Verification items for this drawing (mm, ordinates from the low corner). A direction names the side the tool comes from. Round coordinates to 2 decimals unless told otherwise and drop trailing zeros. Loops run counter-clockwise (first coordinate to the right, second up) from the corner with the lowest first, then second, coordinate; pieces in that order, holes last. Notation, with made-up numbers: (-5, 15.25) - (5, 15.25) arc R25 ccw to (5, 37.25) - close; hole circle Ø11 at (66.25, -6). An arc over 180 degrees is marked (long way). Answer in a Markdown table with one row per item. Add a question column.
(1) Gauge pin test, flat ends, axial feed: pin 1 (0.9 mm diameter, centred on y = 3.5, z = 3, fed in from +X); pin 2 (1.6 mm diameter, centred on x = 0.5, y = 2.5, fed in from +Z); pin 3 (1.8 mm diameter, centred on x = 3, y = 3, fed in from -Z); pin 4 (1 mm diameter, centred on x = 7.5, z = 2.5, fed in from -Y). Record the tip position at first contact, or that the pin passes through.
(2) Cross-section at D-D on x = 4. Enter the section's corners in (y, z), then the cut area to 3 significant figures.
(3) Cross-section at A-A on z = 2.75. Enter the section's corners in (x, y) (3 decimals).
(4) Access from +Z, -Z, +X, -X, +Y, -Y to the whole of each face (thin tool, end or side, straight path). Record for the marked faces 1, 2, 3, 4 and 5.
(5) Thickness scan on line 1 along X through (y, z) = (1.5, 3.25) (3 decimals); line 2 along X through (y, z) = (4.2, 3.5); line 3 along Z through (x, y) = (0.75, 4.35). Record the ranges inside material, lowest first.
(6) Cross-section at C-C on x = 5. Enter the section's corners in (y, z).
(7) Cross-section at B-B on x = 1.1. Enter the section's corners in (y, z) (3 decimals).
(8) Mould release check, pull along X, two halves, no side actions. Record for the marked faces 6, 7, 8 and 9: +X half, -X half, draft (parallel to the pull), parting line (faces both ways), or undercut.
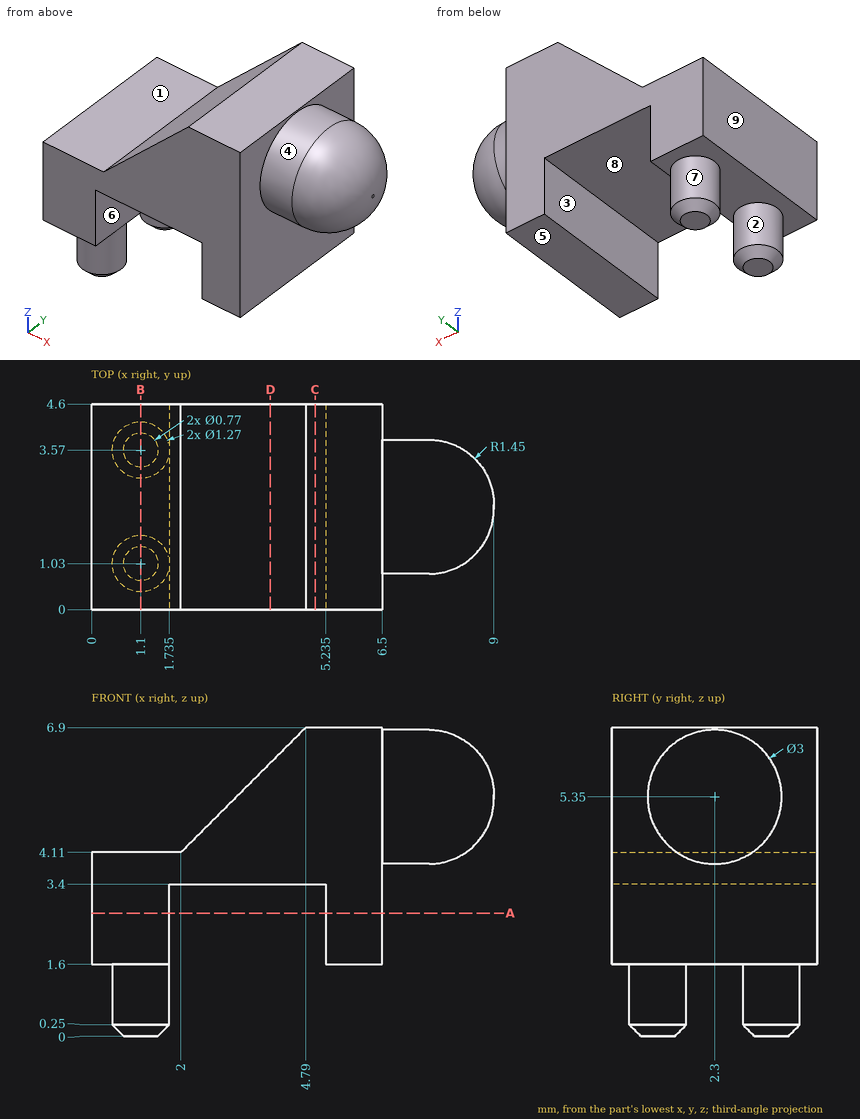
Answers:
| question | item | result |
|---|---|---|
| 1 | pin 1 | stops at x = 6.5 |
| 1 | pin 2 | stops at z = 4.11 |
| 1 | pin 3 | stops at z = 3.4 |
| 1 | pin 4 | passes through |
| 2 | outline | (0, 3.4) - (4.6, 3.4) - (4.6, 6.11) - (0, 6.11) - close |
| 2 | area | 12.5 mm^2 |
| 3 | outline | (0, 0) - (1.735, 0) - (1.735, 4.6) - (0, 4.6) - close; (5.235, 0) - (6.5, 0) - (6.5, 4.6) - (5.235, 4.6) - close |
| 4 | face 1 | +Z, -X, +Y, -Y |
| 4 | face 2 | -Z |
| 4 | face 3 | -Z, +Y, -Y |
| 4 | face 4 | +X |
| 4 | face 5 | -Z, +X, +Y, -Y |
| 5 | line 1 | x = 0 to 1.735, 5.235 to 6.5 |
| 5 | line 2 | x = 0 to 6.5 |
| 5 | line 3 | z = 1.6 to 4.11 |
| 6 | outline | (0, 3.4) - (4.6, 3.4) - (4.6, 6.9) - (0, 6.9) - close |
| 7 | outline | (0, 1.6) - (0.395, 1.6) - (0.395, 0.25) - (0.645, 0) - (1.415, 0) - (1.665, 0.25) - (1.665, 1.6) - (2.935, 1.6) - (2.935, 0.25) - (3.185, 0) - (3.955, 0) - (4.205, 0.25) - (4.205, 1.6) - (4.6, 1.6) - (4.6, 4.11) - (0, 4.11) - close |
| 8 | face 6 | undercut |
| 8 | face 7 | parting line |
| 8 | face 8 | undercut |
| 8 | face 9 | -X half |
